Could you check a few things on this model? Use its own coordinates, in mm. A direction names the side the tool comes from. Round coordinates to 2 decimals unless told otherwise and drop trailing zeros. Loops run counter-clockwise (first coordinate to the right, second up) from the corner with the lowest first, then second, coordinate; pieces in that order, holes last. Notation, with made-up numbers: (26.25, 33.5) -> (61.25, 33.5) arc R8 ccw to (61.25, 48.5) -> close; hole circle Ø8 at (-8, -23.75). An arc over 180 degrees is marked (long way). Write each question's results on one line, items separated by ' | '. Start each with the question number.
1) Imagine slicing it at D-D, the plane x = -78.5. List the corners of the cut face in (y, z) for me (3 decimals), plus the area to 3 significant figures.
2) Imagine slicing it at A-A, the plane z = 0. List the corners of the cut face in (x, y) for me.
3) If I drill on probe 1 along Y at (x, z) = (-1.5, 29); probe 2 along X at (y, z) = (-48, 34.5); probe 3 along X at (y, z) = (47, 0), over which ranges is the centre line in solid material (lowest first)?
4) We'd pull the mould along Z, two halves only. Please class faces 1 (the flat face through (-14, 1, -68.005)), 2 (the flat face through (100.175, -59, 2)), 3 (the cylindrical face through (31.063, 94.806, 22.697)): pulls with the +Z half, pulls with the -Z half, needs draft (parallel to the pull), parting line crosses it, or undercut.
5) Which directions (+Z, -Z, +X, -X, +Y, -Y) give clear straight access to the entire face, cutting with the end or side of a thin tool? Please do faces 4 (the flat face through (47, -16.78, 2)), 5 (the cylindrical face through (-112.68, 48.26, 12.31)), 6 (the cylindrical face through (24.36, -58.597, 28.295)).
6) For P1, Ø2, axis at x = 64.5, z = 26.5, coming from the +Y side; P2, Ø20.5, axis at y = -5, z = 26.5, coming from the +X side, each with a flat end and sliding along its axis, tell me the tip position at first contact or that it passes through.
7) Imagine slicing it at C-C, the plane y = -32. List the corners of the cut face in (x, z) for me (1 decimal), plus the area to 3 significant figures.
8) Imagine slicing it at B-B, the plane x = 62. Give the number of separate pieces and of enclosed holes in the cut face, plus the area to 3 significant figures.
from build123d import *

# Parameters (mm, degrees)
SKETCH1_W                                      = 224.783024271
SKETCH1_H                                      = 138.046096427
BOSS_EXTRUDE1_DEPTH                            = 101.6
SKETCH2_R                                      = 26.66819347
CUT_EXTRUDE1_DEPTH                             = 108.204
SKETCH4_W                                      = 138.046096427
SKETCH4_H                                      = 40.817377809
CUT_EXTRUDE2_DEPTH                             = 108.204
CBORE_FOR_3_4_PAN_HEAD_MACHINE_SCREW1_AT_COUNT = 2
CBORE_FOR_3_4_PAN_HEAD_MACHINE_SCREW1_AT_PITCH = 78.529858642
CBORE_FOR_3_4_PAN_HEAD_MACHINE_SCREW_2_COUNT   = 2
CBORE_FOR_3_4_PAN_HEAD_MACHINE_SCREW_2_PITCH   = 88.813103961
CBORE_FOR_3_4_PAN_HEAD_MACHINE_SCREW_3_COUNT   = 2
CBORE_FOR_3_4_PAN_HEAD_MACHINE_SCREW_3_PITCH   = 46.772278414
CBORE_FOR_3_4_PAN_HEAD_MACHINE_SCREW_4_COUNT   = 2
CBORE_FOR_3_4_PAN_HEAD_MACHINE_SCREW_4_PITCH   = 42.272131605


with BuildPart() as part:
    # Sketch1 → Boss-Extrude1 (new, symmetric)
    with BuildSketch(Plane(origin=(0, 0, 0), x_dir=(1, 0, 0), z_dir=(0, 1, 0))):
        with Locations((-12.21646871, -1.018039059)):
            Rectangle(SKETCH1_W, SKETCH1_H)
    extrude(amount=BOSS_EXTRUDE1_DEPTH, both=True)

    # Sketch2 → Cut-Extrude1 (cut)
    with BuildSketch(Plane(origin=(0, 101.6, 0), x_dir=(1, 0, 0), z_dir=(0, 1, 0))):
        with Locations(Location((-89.023589675, 0, 0), (0, 0, 270))):
            Circle(SKETCH2_R)
    extrude(amount=-CUT_EXTRUDE1_DEPTH, mode=Mode.SUBTRACT)

    # Sketch4 → Cut-Extrude2 (cut)
    with BuildSketch(Plane(origin=(100.175043425, 0, 0), x_dir=(0, 0, -1), z_dir=(1, 0, 0))):
        with Locations((-1.018039059, 3.62821136)):
            Rectangle(SKETCH4_W, SKETCH4_H)
    extrude(amount=-CUT_EXTRUDE2_DEPTH, mode=Mode.SUBTRACT)

    # Sketch7 → CBORE for 3/4 Pan Head Machine Screw1 (revolve, cut)
    with BuildSketch(Plane(origin=(58.259270804, 101.6, 42.822055049), x_dir=(0, 0, 1), z_dir=(1, 0, 0))):
        Polygon((0, 0), (0, 203.2), (9.92124, 203.2), (9.92124, 13.8684), (10.55624, 13.2334), (18.65376, 13.2334), (18.65376, 0.532828266), (19.28876, 0), align=None)
    cbore_for_3_4_pan_head_machine_screw1 = revolve(axis=Axis((58.259270804, 107.95, 42.822055049), (0, -1, 0)), mode=Mode.SUBTRACT)

    # CBORE for 3/4 Pan Head Machine Screw1 at: CBORE for 3/4 Pan Head Machine Screw1 ×2
    with Locations(*[(0, 0, -i * CBORE_FOR_3_4_PAN_HEAD_MACHINE_SCREW1_AT_PITCH) for i in range(1, CBORE_FOR_3_4_PAN_HEAD_MACHINE_SCREW1_AT_COUNT)]):
        add(cbore_for_3_4_pan_head_machine_screw1, mode=Mode.SUBTRACT)

    # CBORE for 3_4 Pan Head Machine Screw 2: CBORE for 3/4 Pan Head Machine Screw1 ×2
    with Locations(*[Vector(-0.46708054288373707, 0, -0.8842147739432052) * (i * CBORE_FOR_3_4_PAN_HEAD_MACHINE_SCREW_2_PITCH) for i in range(1, CBORE_FOR_3_4_PAN_HEAD_MACHINE_SCREW_2_COUNT)]):
        add(cbore_for_3_4_pan_head_machine_screw1, mode=Mode.SUBTRACT)

    # CBORE for 3_4 Pan Head Machine Screw 3: CBORE for 3/4 Pan Head Machine Screw1 ×2
    with Locations(*[Vector(-0.9962520130083015, 0, -0.08649813048215103) * (i * CBORE_FOR_3_4_PAN_HEAD_MACHINE_SCREW_3_PITCH) for i in range(1, CBORE_FOR_3_4_PAN_HEAD_MACHINE_SCREW_3_COUNT)]):
        add(cbore_for_3_4_pan_head_machine_screw1, mode=Mode.SUBTRACT)

    # CBORE for 3_4 Pan Head Machine Screw 4: CBORE for 3/4 Pan Head Machine Screw1 ×2
    with Locations(*[Vector(-0.9813290988359743, 0, -0.19233616346848256) * (i * CBORE_FOR_3_4_PAN_HEAD_MACHINE_SCREW_4_PITCH) for i in range(1, CBORE_FOR_3_4_PAN_HEAD_MACHINE_SCREW_4_COUNT)]):
        add(cbore_for_3_4_pan_head_machine_screw1, mode=Mode.SUBTRACT)


solid = part.part
Checked values:
1) outline: (-101.6, -68.005) -> (101.6, -68.005) -> (101.6, -24.504) -> (-6.604, -24.504) -> (-6.604, 24.504) -> (101.6, 24.504) -> (101.6, 70.041) -> (-101.6, 70.041) -> close | area: 22,700 mm^2
2) outline: (-124.61, -101.6) -> (100.18, -101.6) -> (100.18, -16.78) -> (-8.03, -16.78) -> (-8.03, 24.04) -> (100.18, 24.04) -> (100.18, 101.6) -> (-62.36, 101.6) -> (-62.36, -6.6) -> (-115.69, -6.6) -> (-115.69, 101.6) -> (-124.61, 101.6) -> close
3) probe 1: -101.6 to -16.78, 24.04 to 88.37 | probe 2: -124.61 to 2.71, 26.7 to 52.86, 63.66 to 100.18 | probe 3: -124.61 to -115.69, -62.36 to 100.18
4) face 1: pulls with the -Z half | face 2: needs draft | face 3: undercut
5) face 4: +Z, -Z, +X | face 5: +Y | face 6: +Y, -Y
6) P1: y = 88.37 | P2: x = -8.03
7) outline: (-124.6, -68) -> (100.2, -68) -> (100.2, 70) -> (-124.6, 70) -> close; hole circle Ø19.8 at (16.8, -35.7); hole (8.4, 29.4) arc R9.9 ccw (long way) to (20.1, 44.1) arc R9.9 ccw (long way) to start; hole circle Ø19.8 at (58.3, -35.7); hole circle Ø19.8 at (58.3, 42.8) | area: 29,700 mm^2
8) separate pieces: 6 | enclosed holes: 0 | area: 16,000 mm^2
